Check sheet for the modelled part. Datum: model origin and axes. Units: mm. A direction names the side the tool comes from. Round coordinates to 2 decimals unless told otherwise and drop trailing zeros. Write each loop counter-clockwise with the first axis right and the second up, starting at its lowest first coordinate (ties: lowest second). Pieces come first, ordered by that corner, then holes. Notation, with made-up numbers: (5.5, 55) - (25.5, 55) arc R8 cw to (25.5, 66) - close; hole circle Ø9 at (78, 8). An arc over 180 degrees is marked (long way). Answer as a JSON object with one key per item and string values. Group by question number.
Item 1: Release check for a two-part mould opening along Z. For faces 1 (the flat face through (0, 0, 36.435)), 2 (the flat face through (1.68, -3.63, 18.47)), 3 (the cylindrical face through (-0.637, -0.24, 18.476)) record: pulls with the +Z half, pulls with the -Z half, needs draft (parallel to the pull), parting line crosses it, or undercut.
Item 2: Sectioned sample at B-B on x = -5.5. Record the boundary of the cut face in (y, z).
Item 3: Gauge pin test, flat ends, axial feed: P1, Ø3, axis at y = -4.5, z = 12.5, coming from the -X side; P2, Ø5, axis at x = -5, z = 8.5, coming from the +Y side; P3, Ø1.5, axis at x = 2.5, z = 7.5, coming from the -Y side. Record the tip position at first contact, or that the pin passes through.
Item 4: Set-up check for faces 4 (the flat face through (-1.755, 3.595, 18.473)), 5 (the flat face through (0, 0, -1)), 6 (the flat face through (3, 2, 0)): record each of +Z, -Z, +X, -X, +Y, -Y from which the full face is reachable in a straight line by a thin tool's end or side.
Item 5: Thickness scan on line 1 (Z direction, x = 5, y = -2.75); line 2 (Y direction, x = 2, z = 17.5); line 3 (Y direction, x = 1.5, z = 3.5). Record the ranges inside material, lowest first.
Item 6: Sectioned sample at A-A on z = 25. Record the boundary of the cut face in (x, y), plus the area to 3 significant figures.
Autodesk Inventor part; units mm, degrees
ref_plane "YZ Plane" through (0, 0, 0) normal (1, 0, 0) x (0, 1, 0)
ref_plane "XZ Plane" through (0, 0, 0) normal (0, 1, 0) x (-1, 0, 0)
ref_plane "XY Plane" through (0, 0, 0) normal (0, 0, 1) x (1, 0, 0)
ref_plane "Work Plane3" through (-15.3296, -7.279, -15.06) normal (0.4289346, -0.9033355, 0) x (0.9033355, 0.4289346, 0)
ref_plane "Work Plane1" through (4.8151, 29.7955, -15.06) normal (-0.4289346, 0.9033355, 0) x (-0.9033355, -0.4289346, 0)
ref_plane "Work Plane2" through (-4.6706, -29.7269, -15.06) normal (0.4289346, -0.9033355, 0) x (0.9033355, 0.4289346, 0)
sketch "Sketch1" plane through (-15.3296, -7.279, -15.06) normal (0.4289346, -0.9033355, 0) x (0.9033355, 0.4289346, 0)
  circle A0 centre (16.97, 33.03) radius 7.5
  line L0 (9.47, 15.06) -> (24.47, 15.06)
  arc A1 (20.0714, 51.4951) -> (20.0714, 15.06) centre (87.3367, 33.2775) ccw
  line L1 (20.0714, 15.06) -> (20.0714, 51.4951) construction
  line L2 (20.0714, 15.06) -> (56.5065, 15.06) construction
  line L3 (20.0714, 51.4951) -> (16.97, 51.4951)
  line L4 (16.97, 51.4951) -> (16.97, 15.06)
  line L5 (20.0714, 15.06) -> (16.97, 15.06)
  dimension "d0" = 90
extrude "Extrusion1" add sketch "Sketch1" along normal mid plane 8 contours A1 A0 L4 | A0 L4 L3 A1 | A1 L0 L4 A0
ref_plane "Work Plane4" through (0, 0, 0) normal (0, 0, 1) x (1, 0, 0)
sketch "Sketch2" plane through (0, 0, 0) normal (0, 0, 1) x (1, 0, 0)
  circle A0 centre (0, 0) radius 7.5
  point P0 (0, 0)
extrude "Extrusion2" add sketch "Sketch2" against normal blind 1
mirror "Mirror1" about plane through (0, 0, 36.4351) normal (-0.9033355, -0.4289346, 0) of "Extrusion1"
properties part number "00_lightshit_ray1"
Completed:
{
 "1": {"face 1": "pulls with the +Z half", "face 2": "needs draft", "face 3": "undercut"},
 "2": {"outline": "(-5.1, -1) - (5.1, -1) - (5.1, 0) - (-5.1, 0) - close"},
 "3": {"P1": "x = 0.4", "P2": "y = 3.24", "P3": "y = -3.6"},
 "4": {"face 4": "+Z, -X, +Y", "face 5": "-Z, +X, -X, +Y, -Y", "face 6": "+Z"},
 "5": {"line 1": "-1 to 0", "line 2": "-3.48 to -2.62", "line 3": "-3.72 to 2.09"},
 "6": {"outline": "(-2.63, 3.18) - (0.8, -4.05) - (2.63, -3.18) - (-0.8, 4.05) - close", "area": "16.1 mm²"}
}
